Autodesk Inventor part; units mm, degrees
ref_plane "YZ Plane" through (0, 0, 0) normal (1, 0, 0) x (0, 1, 0)
ref_plane "XZ Plane" through (0, 0, 0) normal (0, 1, 0) x (-1, 0, 0)
ref_plane "XY Plane" through (0, 0, 0) normal (0, 0, 1) x (1, 0, 0)
sketch "Body Outline" plane through (0, 0, 0) normal (0, 1, 0) x (-1, 0, 0)
  line L0 (50, -22.5) -> (-50, -22.5)
  line L1 (-50, -22.5) -> (-50, 22.5)
  line L2 (-50, 22.5) -> (50, 22.5)
  line L3 (50, 22.5) -> (50, -22.5)
  point P0 (0, 0)
  dimension "d0" = 45
  dimension "d1" = 22.5
  dimension "d2" = 100
  dimension "d3" = 50
extrude "Body" add sketch "Body Outline" along normal blind 53
shell "Shell" thickness 5 removed faces 1 at (-16.6667, 53, 7.5)
fillet "Shell Fillet" radius 10 4 edges at (-45, 29, -17.5) (45, 29, -17.5) (45, 29, 17.5) (-45, 29, 17.5)
fillet "Shell Fillet" radius 5 2 edges at (-50, 26.5, -22.5) (50, 26.5, -22.5)
sketch "Lid Fastening Hole Pattern" plane through (0, 53, 0) normal (0, 1, 0) x (1, 0, 0)
  line L0 (45, 22.5) -> (-45, 22.5)
  line L1 (-50, 17.5) -> (-50, -22.5)
  point P0 (0, 0)
  point P1 (-45, 17.5)
  point P2 (45, 17.5)
  point P3 (-45, -17.5)
  point P4 (45, -17.5)
  dimension "d115" = 5
  dimension "d116" = 5
  dimension "d119" = 90
  dimension "d122" = 35
hole "Lid Fastening Holes" at (-45, 53, -17.5) at (45, 53, -17.5) at (-45, 53, 17.5) at (45, 53, 17.5) direction (0, -1, 0) diameter 4.134 depth 14.2 tip angle 118
sketch "Cable Exit Hole Position" plane through (-50, 0, 22.5) normal (0, 0, 1) x (1, 0, 0)
  line L0 (100, 0) -> (0, 0)
  line L1 (100, 0) -> (100, 53)
  point P0 (50, 0)
  point P1 (75, 30)
  dimension "d167" = 30
  dimension "d168" = 25
hole "Cable Exit Hole" at (25, 30, 22.5) direction (0, 0, -1) diameter 15 depth 5
sketch "Flanges Outline" plane through (-50, 0, 22.5) normal (0, 0, 1) x (1, 0, 0)
  line L0 (-19.5, 40) -> (0, 40)
  line L1 (0, 40) -> (0, 20)
  line L2 (0, 20) -> (-19.5, 20)
  line L3 (-19.5, 20) -> (-19.5, 40)
  line L4 (100, 40) -> (119.5, 40)
  line L5 (119.5, 40) -> (119.5, 20)
  line L6 (119.5, 20) -> (100, 20)
  line L7 (100, 20) -> (100, 40)
  line L8 (0, 0) -> (0, 53)
  line L9 (100, 0) -> (100, 53)
  line L10 (100, 0) -> (0, 0)
  line L11 (0, 53) -> (100, 53)
  point P0 (50, 0)
  dimension "d176" = 0
  dimension "d177" = 0
  dimension "d178" = 19.5
  dimension "d179" = 19.5
  dimension "d180" = 20
  dimension "d181" = 20
  dimension "d182" = 13
  dimension "d183" = 13
extrude "Flanges" add sketch "Flanges Outline" against normal blind 9.53 contours L0 L1 L2 L3 | L4 L5 L6 L7
fillet "Flanges Fillet" radius 7 8 edges at (-50, 40, 17.735) (-69.5, 40, 17.735) (-69.5, 20, 17.735) (-50, 20, 17.735) (50, 40, 17.735) (69.5, 40, 17.735) (69.5, 20, 17.735) (50, 20, 17.735)
sketch "Box Fastening Hole Pattern" plane through (-50, 0, 12.97) normal (0, 0, -1) x (-1, 0, 0)
  line L0 (0, 0) -> (0, 53)
  line L1 (-5, 0) -> (-95, 0)
  point P0 (-50, 0)
  point P1 (12.5, 30)
  point P2 (-112.5, 30)
  dimension "d187" = 12.5
  dimension "d188" = 30
  dimension "d191" = 125
hole "Box Fastening Holes" at (-62.5, 30, 12.97) at (62.5, 30, 12.97) direction (0, 0, 1) diameter 6.7 end through all
equation "\"d179\" = d178"
equation "\"d181\" = d180"
properties part number "Connector Box" material "Aluminum 6061"
Can you work these out from the model? Positions are in its coordinate system, mm. A direction names the side the tool comes from. Coordinates: 2 decimals unless noted, no trailing zeros. Order: outer loops, then holes, each group sorted by start corner. A loop starts at its lowest first (then second) coordinate and runs counter-clockwise, first axis right, second up. Notation, with made-up numbers: M 83,-12 L 110,-12 A17 cw 110,5 Z; hole C 11.5,-27.5 d10. An arc over 180 degrees is marked long. Write item = value, one per line.
(1) If we mould it in two halves opening along Z, with no side actions, what happens to faces 4 (the face through (52.1, 42, 17.7)), 5 (the face through (45.4, 37.8, -17.5)), 6 (the face through (-1, 26, -22.5))? For each: pulls with the +Z half, pulls with the -Z half, needs draft (parallel to the pull), parting line crosses it, or undercut.
Results are:
face_4 = needs draft
face_5 = undercut
face_6 = pulls with the -Z half
(2) Suppose I cut it at B-B on x = -21.5. Please give me the cut outline in (y, z).
Results are:
outline = M 0,-22.5 L 53,-22.5 L 53,-17.5 L 5,-17.5 L 5,17.5 L 53,17.5 L 53,22.5 L 0,22.5 Z
(3) Suppose I cut it at A-A on y = 30. State how many separate pieces and enclosed holes the cut face has, plus the area to 3 significant figures.
Results are:
separate_pieces = 3
enclosed_holes = 0
area = 1,590 mm2
(4) Suppose I cut it at D-D on y = 15.5. Please give me the cut outline in (x, z).
Results are:
outline = M -50.46,12.97 L -50,12.97 L -50,-17.5 A5 ccw -45,-22.5 L 45,-22.5 A5 ccw 50,-17.5 L 50,12.97 L 50.46,12.97 L 50.46,22.5 L -50.46,22.5 Z; hole M -45,-7.5 A10 ccw -35,-17.5 L 35,-17.5 A10 ccw 45,-7.5 L 45,7.5 A10 ccw 35,17.5 L -35,17.5 A10 ccw -45,7.5 Z
(5) For faces 1 (the face through (-58, 30, 12.97)), 2 (the face through (44.38, 45.8, 19.47)), 3 (the face through (-52, 42.1, 17.7)), which set-ups out of +Z, -Z, +X, -X, +Y, -Y let a thin tool reach every point of the face, with its end or its side?
Results are:
face_1 = -Z, -X, +Y, -Y
face_2 = +Y
face_3 = +Z, -Z, -X, +Y
(6) I need wall thicknesses on line 1 along X through (y, z) = (30, 20); line 2 along Z through (x, y) = (-19, 28); line 3 along X through (y, z) = (14, 2). Which ranges of each line are inside material? Lowest first, please. Write a range as [from, to].
Results are:
line_1 = [-69.5, -65.85], [-59.15, 17.5], [32.5, 59.15], [65.85, 69.5]
line_2 = [-22.5, -17.5], [17.5, 22.5]
line_3 = [-50, -45], [45, 50]
(7) Suppose I cut it at C-C on z = -6. Please give me the cut outline in (x, y).
Results are:
outline = M -50,0 L 50,0 L 50,53 L 45,53 L 45,5 L -45,5 L -45,53 L -50,53 Z
(8) For pin 1 Ø10.5 at (x, y) = (62.5, 30) entering from -Z; pin 2 Ø4.5 at (y, z) = (26.5, 1.5) entering from -X; pin 3 Ø12 at (y, z) = (17, 2.5) entering from +X; pin 4 Ø5.5 at (x, y) = (-62.5, 30) entering from -Z, each with a flat end and sliding along its axis, tell me the tip position at first contact or that it passes through.
Results are:
pin_1 = 12.97
pin_2 = -50
pin_3 = 50
pin_4 = through
